Input: part model. Units: mm. Frame: model coordinates. Face numbers are marked on the shaded views. Round coordinates to 2 decimals unless told otherwise and drop trailing zeros. Order: outer loops, then holes, each group sorted by start corner. A loop starts at its lowest first (then second) coordinate and runs counter-clockwise, first axis right, second up. Notation, with made-up numbers: M -32,4.5 L 26,4.5 A18 cw 26,26.5 Z; hole C 15,52.25 d4. An arc over 180 degrees is marked long. One line per question, with ' | ' between items.
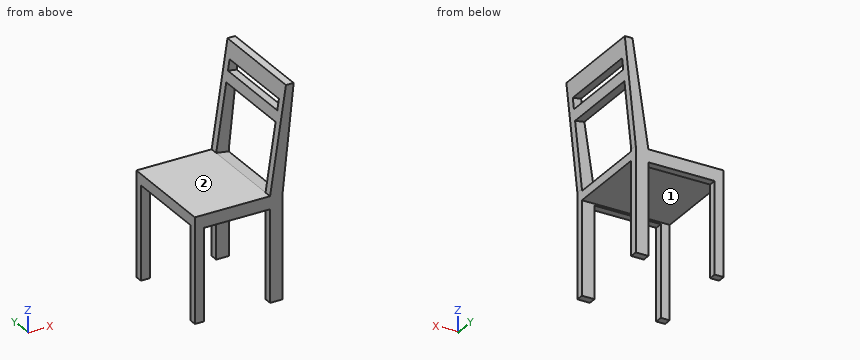
```python
from build123d import *

# Parameters (mm, degrees)
F0_W     = 450
F0_H     = 450
F1_DEPTH = 950
F2_W     = 50
F2_H     = 58.0840170383
F2_H_2   = 416.9159829617
F2_W_2   = 301.8988892436
F3_DEPTH = 450.001
F4_W     = 380
F4_H     = 425
F5_DEPTH = 400.001
F6_W     = 380
F6_H     = 50
F6_H_2   = 305.4825048688
F7_DEPTH = 177.7040327035


with BuildPart() as f1:
    # F0 (on Top) → F1 (new body)
    with BuildSketch(Plane.XY):
        Rectangle(F0_W, F0_H)
    extrude(amount=F1_DEPTH)

    # F2 (on face) → F3 (cut, through all)
    with BuildSketch(Plane.XZ.offset(225)):
        with Locations((200, 445.9579914808)):
            Rectangle(F2_W, F2_H)
        Polygon((-225, 475), (117.622949183, 475), (190, 950), (-225, 950), align=None)
        Polygon((175, 475), (225, 475), (225, 950), align=None)
        with Locations((200, 208.4579914808)):
            Rectangle(F2_W, F2_H_2)
        with Locations((-33.3264954388, 208.4579914808)):
            Rectangle(F2_W_2, F2_H_2)
    extrude(amount=-F3_DEPTH, mode=Mode.SUBTRACT)

    # F4 (on face) → F5 (cut, through all)
    with BuildSketch(Plane.YZ.offset(175)):
        with Locations((0, 212.5)):
            Rectangle(F4_W, F4_H)
    extrude(amount=-F5_DEPTH, mode=Mode.SUBTRACT)

    # F6 (on face) → F7 (cut, through all)
    with BuildSketch(Plane(origin=(44.2192403008, 0, -6.7378067418), x_dir=(0, -1, 0), z_dir=(-0.9885895848, 0, 0.1506341024))):
        with Locations((0, 867.780585023)):
            Rectangle(F6_W, F6_H)
        with Locations((0, 640.0393325886)):
            Rectangle(F6_W, F6_H_2)
    extrude(amount=-F7_DEPTH, mode=Mode.SUBTRACT)


solid = f1.part
```
Item 1: Line query: line 1 along Y through (x, z) = (-192, 117); line 2 along Z through (x, y) = (-98, -197); line 3 along X through (y, z) = (183.5, 457). Output: solid intervals per line, ascending. Write a range as from..to.
Report:
line 1: -225..-190, 190..225 | line 2: 416.92..475 | line 3: -225..175
Item 2: Section query B-B, the plane y = 162. Return loops of the section in (x, z), plus the area to 3 significant figures.
Report:
outline: M -225,425 L 175,425 L 175,466.26 L 117.62,475 L -225,475 Z; M 163.64,777 L 206.11,770.53 L 211.35,820.3 L 171.17,826.43 Z; M 178.7,875.86 L 216.59,870.08 L 225,950 L 190,950 Z | area: 24,700 mm²
Item 3: Section query A-A, the plane z = 139.5. Return loops of the section in (x, y).
Report:
outline: M -225,-225 L -184.28,-225 L -184.28,-190 L -225,-190 Z; M -225,190 L -184.28,190 L -184.28,225 L -225,225 Z; M 117.62,-225 L 175,-225 L 175,-190 L 117.62,-190 Z; M 117.62,190 L 175,190 L 175,225 L 117.62,225 Z
Item 4: Mould query, pull axis Y, two halves, no side actions, for the marked faces 1 and 2. Classes: +Y half, -Y half, draft (parallel to the pull), parting line (faces both ways), or undercut.
Report:
face 1: undercut | face 2: draft
Item 5: Section query C-C, the plane z = 533. Return loops of the section in (x, y), plus the area to 3 significant figures.
Report:
outline: M 126.46,-225 L 181.11,-225 L 181.11,-190 L 126.46,-190 Z; M 126.46,190 L 181.11,190 L 181.11,225 L 126.46,225 Z | area: 3,830 mm²
Item 6: First-contact query: pin 1 (6 mm diameter, centred on x = -22, y = 32.5, fed in from -Z); pin 2 (17.5 mm diameter, centred on x = -87, y = -205, fed in from -Z); pin 3 (10.5 mm diameter, centred on y = -208.5, z = 207.5, fed in from +X). Flat tips, straight axial feed; report the tip coordinate or a pass-through.
Report:
pin 1: z = 425 | pin 2: z = 416.92 | pin 3: x = 175
Item 7: Section query D-D, the plane x = -18. Return loops of the section in (y, z).
Report:
outline: M -225,416.92 L -190,416.92 L -190,425 L 190,425 L 190,416.92 L 225,416.92 L 225,475 L -225,475 Z
